Input: part model. Units: mm. Frame: model coordinates. Coordinates: 2 decimals unless noted, no trailing zeros. Write each loop counter-clockwise with the first axis right and the second up, starting at its lowest first coordinate (ties: lowest second). Pieces come first, ordered by that corner, then holes. Notation, with made-up numbers: (35, 58) - (92, 58) arc R24 ccw to (92, 90) - close; hole circle Ø6 at (29, 25.25). An arc over 180 degrees is marked (long way). Use a Markdown table: item, result. Add a question column.
Q1. Material intervals for probe 1 along Y at (x, z) = (-467, -215.9); probe 2 along Y at (x, z) = (-458.25, -212.5); probe 3 along Z at (x, y) = (-460, 73.5), sorted ascending. Write a range as from..to.
Q2. Pin query (flat end, axial travel): P1, Ø6, axis at x = -467, z = 11.5, coming from the -Y side. Return the tip coordinate at first contact, or that it passes through.
Q3. Section query A-A (y = 63.5). Return the cut outline in (x, z).
Q4. Section query B-B (z = -215.9). Return the cut outline in (x, y), then the cut area to 4 significant figures.
Q5. Mould query, pull axis Z, two halves, no side actions, for faces 1 (the face through (-466.858, 48.044, -236.057)), 2 (the face through (-466.858, 603.854, -221.406)), 3 (the face through (-476.25, 341, -5)), 4 (the face through (-467, 341, 279.4)). Classes: released by +Z, released by -Z, zero draft, split by the parting line, or undercut.
from build123d import *

# Parameters (mm, degrees)
SKETCH1_W           = 19.05
SKETCH1_H           = 577.85
BOSS_EXTRUDE1_DEPTH = 692.15
SKETCH2_R           = 25.4
CUT_EXTRUDE1_DEPTH  = 754.993983729


with BuildPart() as part:
    # Sketch1 → Boss-Extrude1 (new body)
    with BuildSketch(Plane(origin=(0, 0, 0), x_dir=(1, 0, 0), z_dir=(0, 1, 0))):
        with Locations((-466.725, 9.525)):
            Rectangle(SKETCH1_W, SKETCH1_H)
    extrude(amount=BOSS_EXTRUDE1_DEPTH)

    # Sketch2 → Cut-Extrude1 (cut, through all)
    with BuildSketch(Plane.ZY.offset(476.25)):
        with Locations((-215.9, 628.65)):
            Circle(SKETCH2_R)
        with Locations((-215.9, 63.5)):
            Circle(SKETCH2_R)
    extrude(amount=-CUT_EXTRUDE1_DEPTH, mode=Mode.SUBTRACT)


solid = part.part
Values follow:
| question | item | result |
|---|---|---|
| 1 | probe 1 | 0..38.1, 88.9..603.25, 654.05..692.15 |
| 1 | probe 2 | 0..38.33, 88.67..603.48, 653.82..692.15 |
| 1 | probe 3 | -298.45..-239.25, -192.55..279.4 |
| 2 | P1 | y = 0 |
| 3 | outline | (-476.25, -298.45) - (-457.2, -298.45) - (-457.2, -241.3) - (-476.25, -241.3) - close; (-476.25, -190.5) - (-457.2, -190.5) - (-457.2, 279.4) - (-476.25, 279.4) - close |
| 4 | outline | (-476.25, 0) - (-457.2, 0) - (-457.2, 38.1) - (-476.25, 38.1) - close; (-476.25, 88.9) - (-457.2, 88.9) - (-457.2, 603.25) - (-476.25, 603.25) - close; (-476.25, 654.05) - (-457.2, 654.05) - (-457.2, 692.15) - (-476.25, 692.15) - close |
| 4 | area | 11,250 mm2 |
| 5 | face 1 | undercut |
| 5 | face 2 | undercut |
| 5 | face 3 | zero draft |
| 5 | face 4 | released by +Z |
